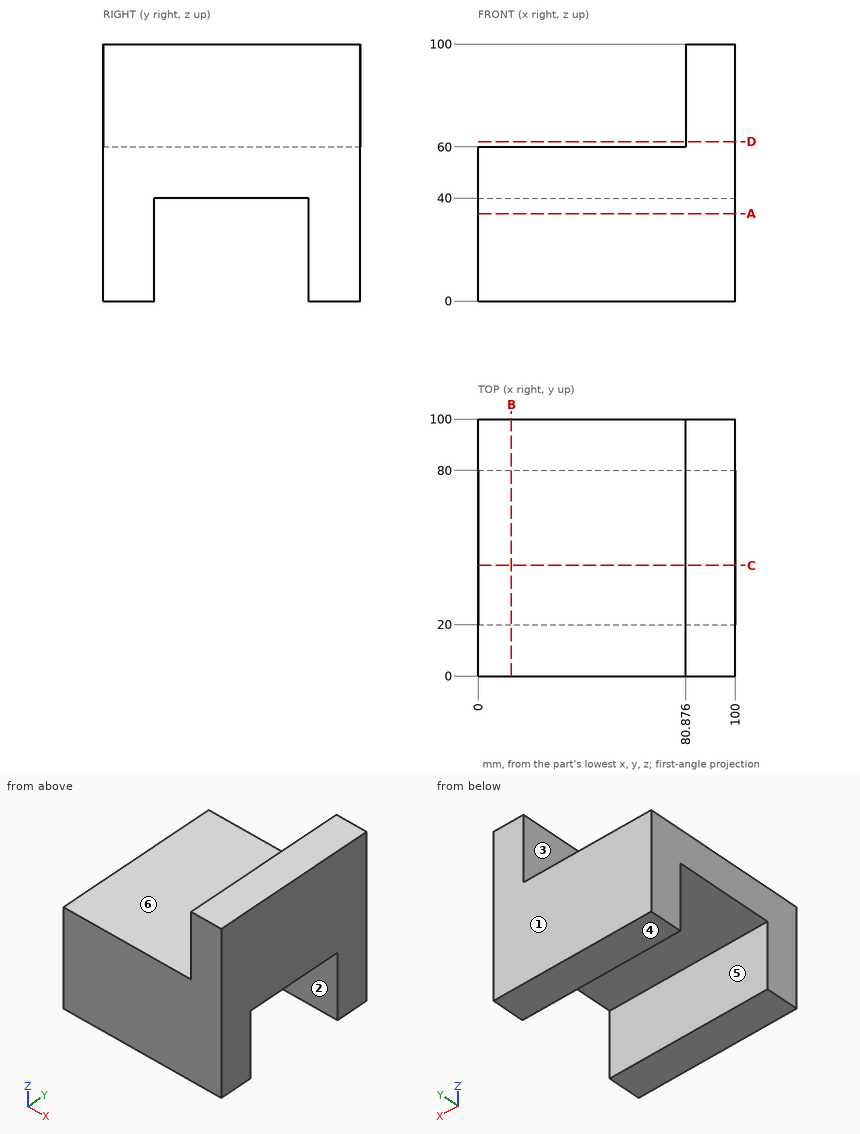
Input: dimensioned drawing with shaded views. Units: mm. Origin: part minimum x, y, z. A direction names the side the tool comes from. Round coordinates to 2 decimals unless told otherwise and drop trailing zeros. Order: outer loops, then holes, each group sorted by start corner. A loop starts at its lowest first (then second) coordinate and runs counter-clockwise, first axis right, second up.
1. Cut plane B-B, the plane x = 13. Output: boundary loops of the cut face in (y, z), then the cut area to 3 significant figures.
The answers:
outline: (0, 0) - (20, 0) - (20, 40) - (80, 40) - (80, 0) - (100, 0) - (100, 60) - (0, 60) - close
area: 3,600 mm2
2. Cut plane A-A, the plane z = 34. Output: boundary loops of the cut face in (x, y).
The answers:
outline: (0, 0) - (100, 0) - (100, 20) - (0, 20) - close; (0, 80) - (100, 80) - (100, 100) - (0, 100) - close
3. Cut plane D-D, the plane z = 62. Output: boundary loops of the cut face in (x, y) (1 decimal), then the cut area to 3 significant figures.
The answers:
outline: (80.9, 0) - (100, 0) - (100, 100) - (80.9, 100) - close
area: 1,910 mm2
4. Cut plane C-C, the plane y = 43. Output: boundary loops of the cut face in (x, z) (1 decimal).
The answers:
outline: (0, 40) - (100, 40) - (100, 100) - (80.9, 100) - (80.9, 60) - (0, 60) - close
5. Pin query (flat end, axial travel): P1, Ø1.5, axis at x = 20, y = 89, coming from the -Z side; P2, Ø12, axis at y = 63, z = 74, coming from the -X side. Return the tip coordinate at first contact, or that it passes through.
The answers:
P1: stops at z = 0
P2: stops at x = 80.88
6. Mould query, pull axis Y, two halves, no side actions, for the marked faces 1, 2 and 3. Classes: released by +Y, released by -Y, zero draft, split by the parting line, or undercut.
The answers:
face 1: released by +Y
face 2: undercut
face 3: zero draft
7. Set-up query: the marked faces 4, 5 and 6. Return all of +Z, -Z, +X, -X, +Y, -Y with unobstructed straight access to the full face (end or side cutting, diameter ignored); none if empty.
The answers:
face 4: -Z, +X, -X, +Y, -Y
face 5: -Z, +X, -X
face 6: +Z, -X, +Y, -Y
8. Material intervals for line 1 (Y direction, x = 80.5, z = 7); line 2 (X direction, y = 21, z = 67) (1 decimal); line 3 (Z direction, x = 53, y = 33), sorted ascending.
The answers:
line 1: y = 0 to 20, 80 to 100
line 2: x = 80.9 to 100
line 3: z = 40 to 60
